from build123d import *

# Parameters (mm, degrees)
BOSS_EXTRUDE1_START = 7
SKETCH2_R           = 2
BOSS_EXTRUDE1_DEPTH = 18
SKETCH3_R           = 10
BOSS_EXTRUDE2_DEPTH = 14
SKETCH4_R           = 8.5
SKETCH4_R_2         = 4
CUT_EXTRUDE1_DEPTH  = 0.5


with BuildPart() as part:
    # Sketch1 → Revolve1 (revolve)
    with BuildSketch(Plane.XY, mode=Mode.PRIVATE) as revolve1_sk:
        Polygon((0, 12), (2.5, 12), (2.5, 11), (2, 11), (2, 0), (0, 0), align=None)
    revolve(revolve1_sk.sketch.rotate(Axis((0, 0, 0), (0, 1, 0)), 90), axis=Axis((0, 0, 0), (0, 1, 0)))

    # Sketch2 → Boss-Extrude1 (add)
    with BuildSketch(Plane.XZ.offset(BOSS_EXTRUDE1_START)):
        with Locations(Location((0, 0, 0), (0, 0, 270))):
            Circle(SKETCH2_R)
    extrude(amount=-BOSS_EXTRUDE1_DEPTH)

    # Sketch3 → Boss-Extrude2 (add)
    with BuildSketch(Plane.XZ.offset(7)):
        with Locations(Location((0, 0, 0), (0, 0, 270))):
            Circle(SKETCH3_R)
    extrude(amount=BOSS_EXTRUDE2_DEPTH)

    # Sketch4 → Cut-Extrude1 (cut)
    with BuildSketch(Plane.XZ.offset(21)):
        with Locations(Location((0, 0, 0), (0, 0, 270))):
            Circle(SKETCH4_R)
        with Locations(Location((0, 0, 0), (0, 0, 270))):
            Circle(SKETCH4_R_2, mode=Mode.SUBTRACT)
    extrude(amount=-CUT_EXTRUDE1_DEPTH, mode=Mode.SUBTRACT)


solid = part.part
Geometry check sheet. Reference: the model listing, model coordinates, mm. A direction names the side the tool comes from. Give positions to 0.01 mm unless a question says otherwise; leave off trailing zeros. Loops run counter-clockwise (first coordinate to the right, second up) from the corner with the lowest first, then second, coordinate; pieces in that order, holes last.
(1) Section check D-D on z = 3.5. Record the cut outline in (x, y), then the cut area to 3 significant figures.
From the geometry:
outline: (-9.37, -21) - (-7.75, -21) - (-7.75, -20.5) - (-1.94, -20.5) - (-1.94, -21) - (1.94, -21) - (1.94, -20.5) - (7.75, -20.5) - (7.75, -21) - (9.37, -21) - (9.37, -7) - (-9.37, -7) - close
area: 256 mm2
(2) Section check B-B on x = 0. Record the cut outline in (y, z), then the cut area to 4 significant figures.
From the geometry:
outline: (-21, -10) - (-7, -10) - (-7, -2) - (11, -2) - (11, -2.5) - (12, -2.5) - (12, 2.5) - (11, 2.5) - (11, 2) - (-7, 2) - (-7, 10) - (-21, 10) - (-21, 8.5) - (-20.5, 8.5) - (-20.5, 4) - (-21, 4) - (-21, -4) - (-20.5, -4) - (-20.5, -8.5) - (-21, -8.5) - close
area: 352.5 mm2
(3) Thickness scan on L1, parallel to X at y = -20.75, z = 0; L2, parallel to Y at x = 2.25, z = -1; L3, parallel to Y at x = 7.5, z = -4.5. Record the ranges inside material, lowest first.
From the geometry:
L1: x = -10 to -8.5, -4 to 4, 8.5 to 10
L2: y = -21 to -7, 11 to 12
L3: y = -21 to -7
(4) Section check C-C on y = -5.5. Record the cut outline in (x, z), then the cut area to 3 significant figures.
From the geometry:
outline: circle Ø4 at (0, 0)
area: 12.6 mm2
(5) Section check A-A on z = 0. Record the cut outline in (x, y).
From the geometry:
outline: (-10, -21) - (-8.5, -21) - (-8.5, -20.5) - (-4, -20.5) - (-4, -21) - (4, -21) - (4, -20.5) - (8.5, -20.5) - (8.5, -21) - (10, -21) - (10, -7) - (2, -7) - (2, 11) - (2.5, 11) - (2.5, 12) - (-2.5, 12) - (-2.5, 11) - (-2, 11) - (-2, -7) - (-10, -7) - close
(6) Release check for a two-part mould opening along Z. For faces 4 (the flat face through (-2, -20.5, -4)), 5 (the cylindrical face through (-0.1, 11.5, 2.5)), 6 (the flat face through (0, 12, 0)) record: released by +Z, released by -Z, zero draft, split by the parting line, or undercut.
From the geometry:
face 4: undercut
face 5: split by the parting line
face 6: zero draft
(7) Set-up check for faces 1 (the cylindrical face through (-2, 2, 0)), 2 (the cylindrical face through (8.428, -20.754, 1.107)), 3 (the flat face through (-7.4, -21, 4.5)): record each of +Z, -Z, +X, -X, +Y, -Y from which the full face is reachable in a straight line by a thin tool's end or side.
From the geometry:
face 1: none
face 2: -Y
face 3: +Z, -Z, +X, -X, -Y
(8) Depth check by flat-ended pin: pin 1 Ø2 at (x, z) = (5.5, 3.5) entering from +Y; pin 2 Ø12 at (x, y) = (7, -5.5) entering from -Z; pin 3 Ø3 at (x, z) = (-1, -6) entering from -Y. Enter the tip coordinate at first touch or a pass-through.
From the geometry:
pin 1: stops at y = -7
pin 2: stops at z = -9.93
pin 3: stops at y = -20.5
